Verification items for the finished model (mm, model axes). A direction names the side the tool comes from. Coordinates: 2 decimals unless noted, no trailing zeros. Order: outer loops, then holes, each group sorted by start corner. A loop starts at its lowest first (then second) coordinate and runs counter-clockwise, first axis right, second up. Notation, with made-up numbers: M -20.5,81 L 6.5,81 A19 ccw 6.5,104 Z; hole C -10,-23 d6. An arc over 180 degrees is marked long. Write item = value, one per line.
```python
from build123d import *

# Parameters (mm, degrees)
SKETCH_1_W          = 27
SKETCH_1_H          = 15
EXTRUDE_1_DEPTH     = 1
SKETCH_2_R          = 2.425
CUT_EXTRUDE_1_DEPTH = 16.475787541
EXTRUDE_2_DEPTH     = 15
SKETCH_6_W          = 1.5
SKETCH_6_H          = 2
EXTRUDE_3_DEPTH     = 4
SKETCH_7_R          = 1.35
CUT_EXTRUDE_3_DEPTH = 1.5
FILLET_1_R          = 3
CHAMFER_1_SIZE      = 1
CUT_EXTRUDE_4_REACH = 39.101
SKETCH_8_R          = 2


# Some blends are built 0.0001 mm under size
with BuildPart() as part:
    # 草图1 → 凸台-拉伸1 (new body)
    with BuildSketch(Plane.XY):
        Rectangle(SKETCH_1_W, SKETCH_1_H)
    extrude(amount=EXTRUDE_1_DEPTH)

    # 草图2 → 切除-拉伸1 (cut, through all)
    with BuildSketch(Plane.XY.offset(1)):
        with Locations((0, 4.025)):
            Circle(SKETCH_2_R)
        with Locations((0, -4.025)):
            Circle(SKETCH_2_R)
        with Locations((8.05, 4.025)):
            Circle(SKETCH_2_R)
        with Locations((8.05, -4.025)):
            Circle(SKETCH_2_R)
        with Locations((-8.05, 4.025)):
            Circle(SKETCH_2_R)
        with Locations((-8.05, -4.025)):
            Circle(SKETCH_2_R)
    extrude(amount=-CUT_EXTRUDE_1_DEPTH, mode=Mode.SUBTRACT)

    # 草图3 → 凸台-拉伸2 (add)
    with BuildSketch(Plane.XZ.offset(7.5)):
        Polygon((13.5, 0), (19, 0), (19, -28.5), (-4.5, -28.5), (-4.5, -30), (20.5, -30), (20.5, 1), (13.5, 1), align=None)
    extrude(amount=-EXTRUDE_2_DEPTH)

    # 草图6 → 凸台-拉伸3 (add, symmetric)
    with BuildSketch(Plane(origin=(0, 0, 0), x_dir=(1, 0, 0), z_dir=(0, 1, 0))):
        Polygon((19, 0), (19, 5), (14, 0), align=None)
        Polygon((19, 28.5), (14, 28.5), (19, 23.5), align=None)
        with Locations((18.25, 20)):
            Rectangle(SKETCH_6_W, SKETCH_6_H)
    extrude(amount=EXTRUDE_3_DEPTH, both=True)

    # 草图7 → 切除-拉伸3 (cut)
    with BuildSketch(Plane(origin=(0, 0, -30), x_dir=(-1, 0, 0), z_dir=(0, 0, -1))):
        with BuildLine():
            ThreePointArc((4.5, 0), (3.401301202, -2.946379157), (0.641711051, -4.454010207))
            Line((0.641711051, -4.454010207), (-20.5, -7.5))
            Line((-20.5, -7.5), (4.5, -7.5))
            Line((4.5, -7.5), (4.5, 0))
        make_face()
        with BuildLine():
            Line((-20.5, 7.5), (0.641711051, 4.454010207))
            ThreePointArc((0.641711051, 4.454010207), (3.401301202, 2.946379157), (4.5, 0))
            Line((4.5, 0), (4.5, 7.5))
            Line((4.5, 7.5), (-20.5, 7.5))
        make_face()
        Circle(SKETCH_7_R)
    extrude(amount=-CUT_EXTRUDE_3_DEPTH, mode=Mode.SUBTRACT)

    # 圆角1
    # the kernel refuses this fillet: 3 mm, written as the material it adds along each edge
    with BuildSketch(Plane(origin=(19, -3.5, -28.5), x_dir=(-1, 0, 0), z_dir=(0, 1, 0))) as fillet_1_piece_1_section:
        with BuildLine():
            CenterArc((FILLET_1_R, FILLET_1_R), FILLET_1_R, 180, 90)
            Line((0, FILLET_1_R), (0, 0))
            Line((0, 0), (FILLET_1_R, 0))
        make_face()
    fillet_1_piece_1 = extrude(amount=18.283887658, mode=Mode.PRIVATE)
    fillet_1_piece_1 = split(fillet_1_piece_1, bisect_by=Plane(origin=(18.119115161, 7.156974268, -27.821481802), z_dir=(0.1426024558755584, -0.9897800460598605, 0)), keep=Keep.TOP, mode=Mode.PRIVATE)
    add(fillet_1_piece_1)
    with BuildSketch(Plane(origin=(19, -3.5, 0), x_dir=(0, 0, -1), z_dir=(0, 1, 0)), Plane(origin=(19, -7.5, 0), x_dir=(0, 0, -1), z_dir=(0, 1, 0))) as fillet_1_piece_2:
        with BuildLine():
            CenterArc((FILLET_1_R, FILLET_1_R), FILLET_1_R, 180, 90)
            Line((0, FILLET_1_R), (0, 0))
            Line((0, 0), (FILLET_1_R, 0))
        make_face()
    extrude(amount=11)
    with BuildSketch(Plane(origin=(19, -14.783887658, -28.5), x_dir=(-1, 0, 0), z_dir=(0, 1, 0))) as fillet_1_piece_3_section:
        with BuildLine():
            CenterArc((FILLET_1_R, FILLET_1_R), FILLET_1_R, 180, 90)
            Line((0, FILLET_1_R), (0, 0))
            Line((0, 0), (FILLET_1_R, 0))
        make_face()
    fillet_1_piece_3 = extrude(amount=18.283887658, mode=Mode.PRIVATE)
    fillet_1_piece_3 = split(fillet_1_piece_3, bisect_by=Plane(origin=(18.119115161, -7.156974268, -27.821481802), z_dir=(0.1426024558755584, 0.9897800460598605, 0)), keep=Keep.TOP, mode=Mode.PRIVATE)
    add(fillet_1_piece_3)
    # the kernel refuses this fillet: 3 mm, written as the material it takes off along each edge
    with BuildSketch(Plane(origin=(20.5, -15, 1), x_dir=(0, 0, -1), z_dir=(0, 1, 0))) as fillet_1_2_piece_1:
        with BuildLine():
            CenterArc((FILLET_1_R, FILLET_1_R), FILLET_1_R, 180, 90)
            Line((0, FILLET_1_R), (0, 0))
            Line((0, 0), (FILLET_1_R, 0))
        make_face()
    extrude(amount=30, mode=Mode.SUBTRACT)
    with BuildSketch(Plane(origin=(20.5, -15, -30), x_dir=(0, 0, 1), z_dir=(0, 1, 0))) as fillet_1_2_piece_2:
        with BuildLine():
            CenterArc((FILLET_1_R, -FILLET_1_R), FILLET_1_R, 90, 90)
            Line((0, -FILLET_1_R), (0, 0))
            Line((0, 0), (FILLET_1_R, 0))
        make_face()
    extrude(amount=30, mode=Mode.SUBTRACT)

    # 倒角1
    chamfer_1_edges = [part.edges().sort_by_distance(p)[0] for p in [
        (-13.5, 0, 0),
    ]]
    chamfer(chamfer_1_edges, length=CHAMFER_1_SIZE - 0.0001)  # a hair under: the kernel refuses the full size

    # 草图8 → 切除-拉伸4 (cut, up to next)
    with BuildSketch(Plane(origin=(0, 0, 0), x_dir=(-1, 0, 0), z_dir=(0, 0, -1)), mode=Mode.PRIVATE) as cut_extrude_4_sk1:
        Circle(SKETCH_8_R)
    cut_extrude_4_tool1 = extrude(cut_extrude_4_sk1.sketch, amount=-CUT_EXTRUDE_4_REACH, mode=Mode.PRIVATE) & part.part
    add(cut_extrude_4_tool1.solids().sort_by_distance((0, 0, 0))[0], mode=Mode.SUBTRACT)


solid = part.part
```
Item 1: Tool access check on faces 4 (the flat face through (17, 0, -3)), 5 (the flat face through (18, -4, -20)), 6 (the cylindrical face through (-2, 0, 0.5)), 7 (the cylindrical face through (18.14, 5.62, -27.6)). Record the directions out of +Z, -Z, +X, -X, +Y, -Y that give a thin tool (end or side, any length) a straight path to the whole face; none if there is none.
Report:
face_4 = -X, +Y, -Y
face_5 = -X, -Y
face_6 = +Z
face_7 = -X, +Y
Item 2: Sectioned sample at C-C, the plane x = 0. Enter the section's corners in (y, z).
Report:
outline = M -7.5,0 L -6.45,0 L -6.45,1 L -7.5,1 Z; M -4.55,-30 L -1.35,-30 L -1.35,-28.5 L -4.55,-28.5 Z; M 1.35,-30 L 4.55,-30 L 4.55,-28.5 L 1.35,-28.5 Z; M 6.45,0 L 7.5,0 L 7.5,1 L 6.45,1 Z
Item 3: Sectioned sample at B-B, the plane y = -6. Give the number of separate pieces and of enclosed holes in the cut face, then the cut area to 3 significant figures.
Report:
separate_pieces = 4
enclosed_holes = 0
area = 83.4 mm^2
Item 4: Sectioned sample at D-D, the plane z = -4. Enter the section's corners in (x, y).
Report:
outline = M 18,-4 L 19,-4 L 19,-7.5 L 20.5,-7.5 L 20.5,7.5 L 19,7.5 L 19,4 L 18,4 Z
Item 5: Gauge pin test, flat ends, axial feed: pin 1 (0.6 mm diameter, centred on y = 1, z = -20, fed in from -X); pin 2 (5 mm diameter, centred on y = 5.5, z = -13.5, fed in from -X); pin 3 (0.8 mm diameter, centred on x = 18, z = -19.5, fed in from -Y). Record the tip position at first contact, or that the pin passes through.
Report:
pin_1 = 17.5
pin_2 = 19
pin_3 = -4
Item 6: Scan lines: L1, parallel to Z at x = 4, y = -3; L2, parallel to X at y = 5, z = -3.5; L3, parallel to Z at x = 4, y = 5.75. Record each from-to range of solid material in increasing order. Write a range as from..to.
Report:
L1 = -30..-28.5, 0..1
L2 = 19..20.5
L3 = 0..1
Item 7: Sectioned sample at A-A, the plane x = -8.05. Enter the section's corners in (y, z), then the cut area to 3 significant figures.
Report:
outline = M -7.5,0 L -6.45,0 L -6.45,1 L -7.5,1 Z; M -1.6,0 L 1.6,0 L 1.6,1 L -1.6,1 Z; M 6.45,0 L 7.5,0 L 7.5,1 L 6.45,1 Z
area = 5.30 mm^2
Item 8: Release check for a two-part mould opening along X. For faces 1 (the flat face through (-13, -0.1, 0.5)), 2 (the flat face through (18, 0, -19)), 3 (the cylindrical face through (7.52, 1.66, 0.51)) record: pulls with the +X half, pulls with the -X half, needs draft (parallel to the pull), parting line crosses it, or undercut.
Report:
face_1 = pulls with the -X half
face_2 = needs draft
face_3 = undercut
